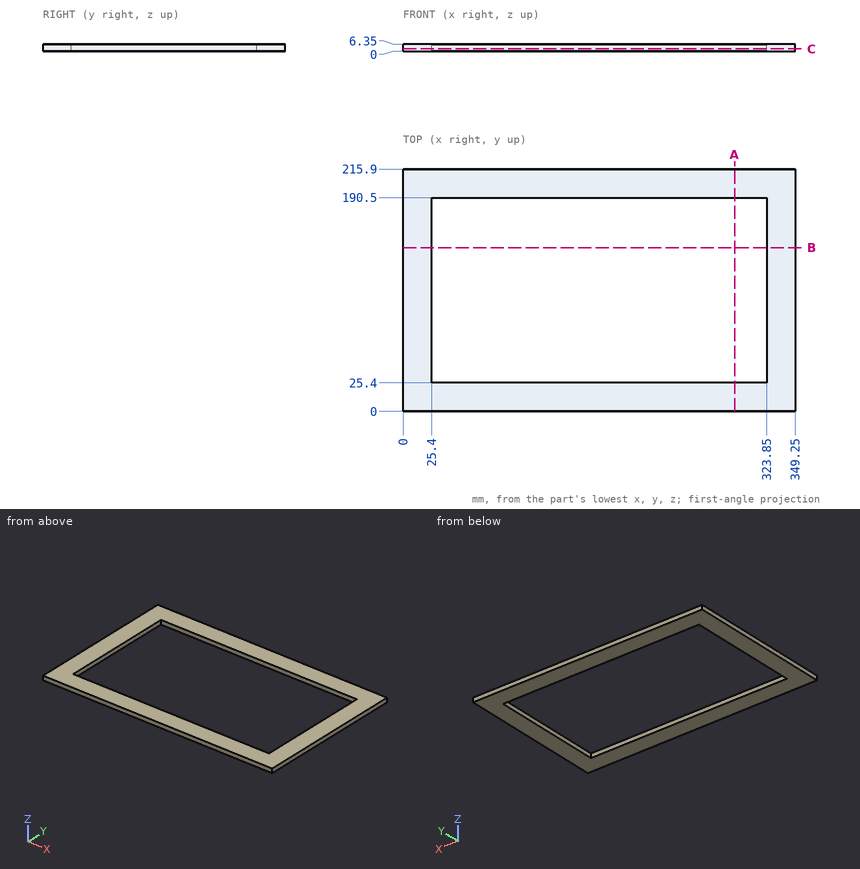
Print and shaded views of the part. All mm, measured from the part's lowest x, y and z. Give positions to 0.01 mm unless a question says otherwise; leave off trailing zeros. Write each loop counter-clockwise with the first axis right and the second up, starting at its lowest first coordinate (ties: lowest second). Pieces come first, ordered by that corner, then holes. Notation, with made-up numbers: M 80,9 L 139,9 A23 ccw 139,31 Z; hole C 57.25,69 d9. An arc over 180 degrees is marked long. Use a Markdown table: item, result.
1) Drill centre lines: line 1 (Y direction, x = 202, z = 1.25); line 2 (X direction, y = 98, z = 4.5). Where is each one in solid material? Low to high. Write a range as from..to.
Responses:
| item | result |
|---|---|
| line 1 | y = 0..25.4, 190.5..215.9 |
| line 2 | x = 0..25.4, 323.85..349.25 |
2) Cut at C-C (z = 2). List the corners of the cut face in (x, y).
Responses:
| item | result |
|---|---|
| outline | M 0,0 L 349.25,0 L 349.25,215.9 L 0,215.9 Z; hole M 25.4,25.4 L 323.85,25.4 L 323.85,190.5 L 25.4,190.5 Z |
3) Cut at A-A (x = 295.5). List the corners of the cut face in (y, z).
Responses:
| item | result |
|---|---|
| outline | M 0,0 L 25.4,0 L 25.4,6.35 L 0,6.35 Z; M 190.5,0 L 215.9,0 L 215.9,6.35 L 190.5,6.35 Z |
4) Cut at B-B (y = 146). List the corners of the cut face in (x, z), and give its area (3 significant figures).
Responses:
| item | result |
|---|---|
| outline | M 0,0 L 25.4,0 L 25.4,6.35 L 0,6.35 Z; M 323.85,0 L 349.25,0 L 349.25,6.35 L 323.85,6.35 Z |
| area | 323 mm2 |
